Could you check a few things on this model? Use its own coordinates, in mm. Face numbers are marked on the shaded views. A direction names the side the tool comes from. Round coordinates to 2 decimals unless told otherwise and drop trailing zeros. Write each loop counter-clockwise with the first axis right and the second up, starting at its lowest first coordinate (ties: lowest second). Pieces come first, ordered by that corner, then holes. Notation, with made-up numbers: (56.5, -1.5) -> (67.5, -1.5) arc R16 cw to (67.5, 5.5) -> close; hole circle Ø6 at (82, 0). An arc over 180 degrees is marked (long way). Answer in a Markdown table with one row per item. Add a question column.
```python
from build123d import *

# Parameters (mm, degrees)
SALIENTE_EXTRUIR1_DEPTH = 100
CROQUIS2_R              = 6.35
CORTAR_EXTRUIR1_DEPTH   = 100


with BuildPart() as part:
    # Croquis1 → Saliente-Extruir1 (new body)
    with BuildSketch(Plane(origin=(0, 0, 0), x_dir=(0, 0, -1), z_dir=(1, 0, 0))):
        with BuildLine():
            Line((8, 0), (100, 0))
            Line((100, 0), (100, 15.875))
            Line((100, 15.875), (8, 15.875))
            ThreePointArc((8, 15.875), (-8.882174401, 8.882174401), (-15.875, -8))
            Line((-15.875, -8), (-15.875, -120))
            Line((-15.875, -120), (0, -120))
            Line((0, -120), (0, -8))
            ThreePointArc((0, -8), (2.343145751, -2.343145751), (8, 0))
        make_face()
    extrude(amount=SALIENTE_EXTRUIR1_DEPTH)

    # Croquis2 → Cortar-Extruir1 (cut)
    with BuildSketch(Plane.XY.offset(15.875)):
        with Locations((15, -34.089894909)):
            Circle(CROQUIS2_R)
        with Locations((85, -34.089894909)):
            Circle(CROQUIS2_R)
        with Locations((15, -105)):
            Circle(CROQUIS2_R)
        with Locations((85, -105)):
            Circle(CROQUIS2_R)
        with Locations((51.532189387, -34.089894909)):
            Circle(CROQUIS2_R)
    extrude(amount=-CORTAR_EXTRUIR1_DEPTH, mode=Mode.SUBTRACT)


solid = part.part
```
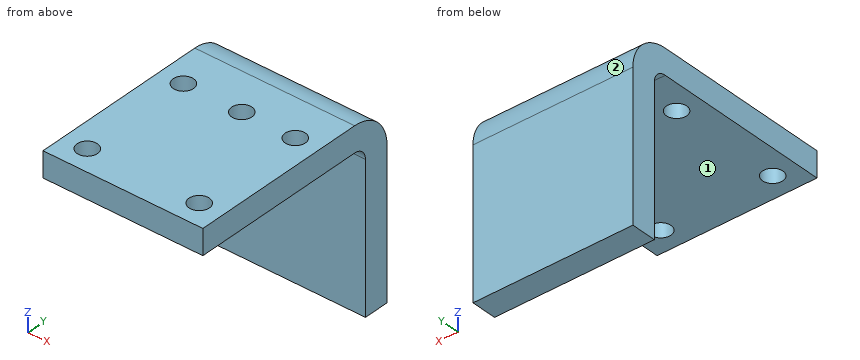
(1) Suppose I cut it at D-D, the plane x = 65.5. Please give me the cut outline in (y, z) (3 decimals), then the cut area to 3 significant figures.
(2) On a 3-axis mill with a long thin cutter (end or side, diameter ignored), from which of +Z, -Z, +X, -X, +Y, -Y can I reach the whole of each face in a straight line? I mean the marked faces 1 and 2. Say none if no direction works.
(3) Suppose I cut it at C-C, the plane x = 53. Please give me the cut outline in (y, z) (3 decimals).
(4) Suppose I cut it at A-A, the plane y = -105. Please give me the cut outline in (x, z) (3 decimals), then the cut area to 3 significant figures.
(5) For P1, Ø4, axis at x = 48, y = -85, coming from the -Z side; P2, Ø4, axis at x = 84.5, z = -71.5, coming from the -Y side, each with a flat end and sliding along its axis, tell me the tip position at first contact or that it passes through.
(6) I need wall thicknesses on L1, parallel to Y at x = 15, z = 3.75; L2, parallel to Y at x = 12, z = -87 (3 decimals); L3, parallel to Y at x = 15, z = 11. Which ranges of each line are inside material? Lowest first, please.
(7) Suppose I cut it at B-B, the plane x = 85. Please give me the cut outline in (y, z) (3 decimals), then the cut area to 3 significant figures.
Response:
| question | item | result |
|---|---|---|
| 1 | outline | (-120, 0) -> (-8, 0) arc R8 cw to (0, -8) -> (0, -100) -> (15.875, -100) -> (15.875, -8) arc R23.875 ccw to (-8, 15.875) -> (-120, 15.875) -> close |
| 1 | area | 3,640 mm² |
| 2 | face 1 | -Z, +X, -X, -Y |
| 2 | face 2 | +Z, +X, -X, +Y |
| 3 | outline | (-120, 0) -> (-40.268, 0) -> (-40.268, 15.875) -> (-120, 15.875) -> close; (-27.912, 0) -> (-8, 0) arc R8 cw to (0, -8) -> (0, -100) -> (15.875, -100) -> (15.875, -8) arc R23.875 ccw to (-8, 15.875) -> (-27.912, 15.875) -> close |
| 4 | outline | (0, 0) -> (8.65, 0) -> (8.65, 15.875) -> (0, 15.875) -> close; (21.35, 0) -> (78.65, 0) -> (78.65, 15.875) -> (21.35, 15.875) -> close; (91.35, 0) -> (100, 0) -> (100, 15.875) -> (91.35, 15.875) -> close |
| 4 | area | 1,180 mm² |
| 5 | P1 | z = 0 |
| 5 | P2 | y = 0 |
| 6 | L1 | -120 to -111.35, -98.65 to -40.44, -27.74 to 12.78 |
| 6 | L2 | 0 to 15.875 |
| 6 | L3 | -120 to -111.35, -98.65 to -40.44, -27.74 to 6.46 |
| 7 | outline | (-120, 0) -> (-111.35, 0) -> (-111.35, 15.875) -> (-120, 15.875) -> close; (-98.65, 0) -> (-40.44, 0) -> (-40.44, 15.875) -> (-98.65, 15.875) -> close; (-27.74, 0) -> (-8, 0) arc R8 cw to (0, -8) -> (0, -100) -> (15.875, -100) -> (15.875, -8) arc R23.875 ccw to (-8, 15.875) -> (-27.74, 15.875) -> close |
| 7 | area | 3,230 mm² |
